Geometry check sheet. Reference: drawing and pictorial views, mm from the part's lowest x, y, z. A direction names the side the tool comes from. Coordinates: 2 decimals unless noted, no trailing zeros. Order: outer loops, then holes, each group sorted by start corner. A loop starts at its lowest first (then second) coordinate and runs counter-clockwise, first axis right, second up. Notation, with made-up numbers: (-19, -16.75) -> (10, -16.75) arc R29 ccw to (10, 10.25) -> close; hole circle Ø4 at (46, 10). An arc over 180 degrees is marked (long way). Use CSV: the item, a comma, the result in double quotes. Start each with the question number.
1) Scan lines: line 1 along X through (y, z) = (11.1, 23); line 2 along Y through (x, z) = (18.5, 17.75). Record each from-to range of solid material in increasing order.
2) Sectioned sample at B-B on x = 2. Record the boundary of the cut face in (y, z), then the cut area to 3 significant figures.
3) Tool access check on the marked faces 1 and 2. Record the directions out of +Z, -Z, +X, -X, +Y, -Y that give a thin tool (end or side, any length) a straight path to the whole face; none if there is none.
4) Sectioned sample at A-A on z = 2. Record the boundary of the cut face in (x, y), then the cut area to 3 significant figures.
5) Sectioned sample at C-C on z = 11.75. Record the boundary of the cut face in (x, y).
6) Go/stop test with flat-tipped pins: pin 1 (1 mm diameter, centred on x = 32.5, y = 7, fed in from -Z); pin 2 (1.6 mm diameter, centred on x = 32, y = 3.5, fed in from +Z); pin 3 (7.5 mm diameter, centred on x = 23, z = 15.5, fed in from -Y). Record where each tip stops, or that it passes through.
7) Sectioned sample at D-D on y = 1.25. Record the boundary of the cut face in (x, z).
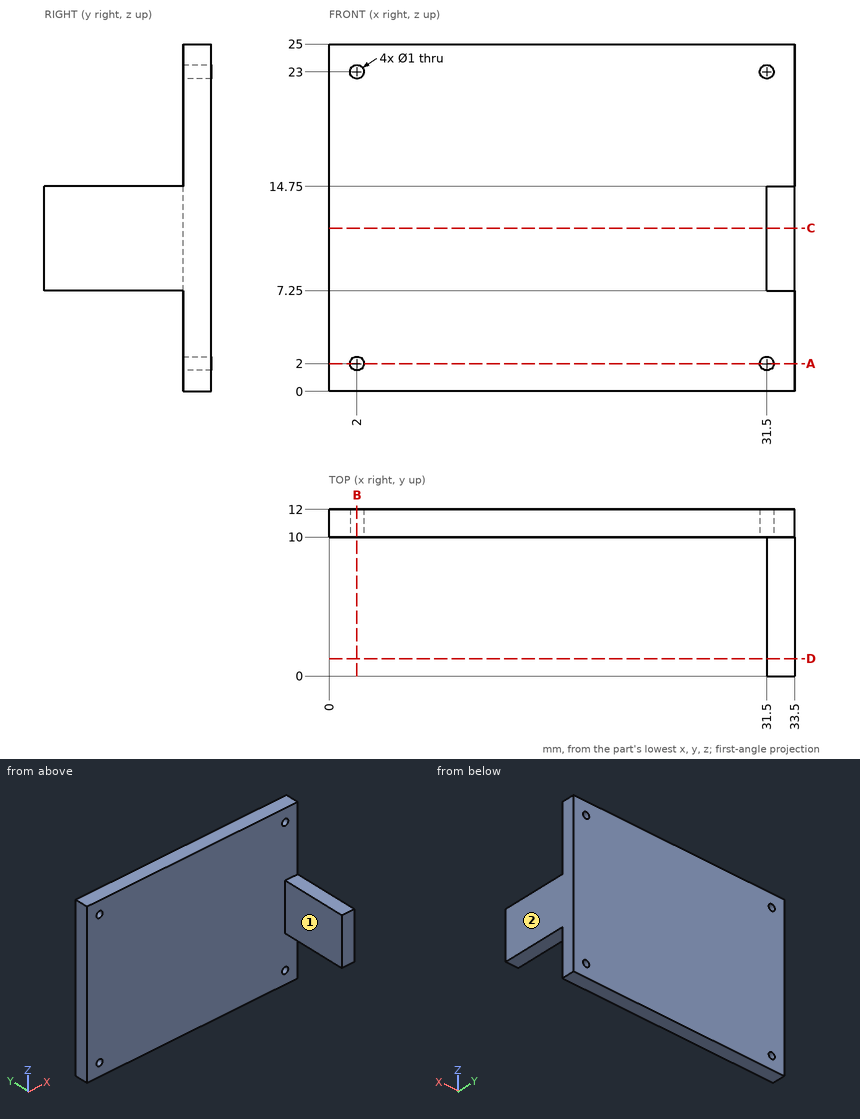
Answers follow:
1,line 1,"x = 0 to 1.5, 2.5 to 31, 32 to 33.5"
1,line 2,"y = 10 to 12"
2,outline,"(10, 0) -> (12, 0) -> (12, 1.5) -> (10, 1.5) -> close; (10, 2.5) -> (12, 2.5) -> (12, 22.5) -> (10, 22.5) -> close; (10, 23.5) -> (12, 23.5) -> (12, 25) -> (10, 25) -> close"
2,area,"46.0 mm²"
3,face 1,"+Z, -Z, -X, -Y"
3,face 2,"+Z, -Z, +X, +Y, -Y"
4,outline,"(0, 10) -> (1.5, 10) -> (1.5, 12) -> (0, 12) -> close; (2.5, 10) -> (31, 10) -> (31, 12) -> (2.5, 12) -> close; (32, 10) -> (33.5, 10) -> (33.5, 12) -> (32, 12) -> close"
4,area,"63.0 mm²"
5,outline,"(0, 10) -> (31.5, 10) -> (31.5, 0) -> (33.5, 0) -> (33.5, 12) -> (0, 12) -> close"
6,pin 1,"stops at z = 7.25"
6,pin 2,"stops at z = 14.75"
6,pin 3,"stops at y = 10"
7,outline,"(31.5, 7.25) -> (33.5, 7.25) -> (33.5, 14.75) -> (31.5, 14.75) -> close"
